from build123d import *

# Parameters (mm, degrees)
F0_R            = 50
F1_DEPTH        = 50
F2_R            = 25
F3_DEPTH        = 50
F5_DEPTH        = 50
F5_COPIES_COUNT = 12


# Not quite as in the source:
# - a pattern or mirror of a feature is missing from the dataset's text; its kind, count and spacing are read off the source's solid


with BuildPart() as f1:
    # F0 (on Top) → F1 (new body)
    with BuildSketch(Plane.XY):
        Circle(F0_R)
    extrude(amount=F1_DEPTH)

    # F2 (on Top) → F3 (cut)
    with BuildSketch(Plane.XY):
        Circle(F2_R)
    extrude(amount=F3_DEPTH, mode=Mode.SUBTRACT)

    # F4 (on Top) → F5 (join)
    with BuildSketch(Plane.XY):
        with BuildLine():
            Line((24.2363690546, 14.6788293603), (23.4842319041, 10.750179179))
            ThreePointArc((23.4842319041, 10.750179179), (35.7966783621, 13.5258846201), (42.1475842595, 24.4330782443))
            Line((42.1475842595, 24.4330782443), (38.1746449562, 24.8975734892))
            ThreePointArc((38.1746449562, 24.8975734892), (33.4316236094, 16.7517982205), (24.2363690546, 14.6788293603))
        make_face()
    f5 = extrude(amount=-F5_DEPTH)

    # F5_copies: F5 ×12 about axis
    f5_copies_axis = Axis((0, 0, 0), (0, 0, 1))
    for i in range(1, F5_COPIES_COUNT):
        add(f5.rotate(f5_copies_axis, i * 360 / F5_COPIES_COUNT))


solid = f1.part
Check sheet for the modelled part. Datum: model origin and axes. Units: mm. A direction names the side the tool comes from. Give positions to 0.01 mm unless a question says otherwise; leave off trailing zeros. Write each loop counter-clockwise with the first axis right and the second up, starting at its lowest first coordinate (ties: lowest second). Pieces come first, ordered by that corner, then holes. Notation, with made-up numbers: (3, 77) -> (9, 77) arc R19 ccw to (9, 112) -> close; hole circle Ø9 at (40.5, 50). An arc over 180 degrees is marked (long way). One line per item, written item: value. Start each with the question number.
Item 1: Section check C-C on z = -32. State how many separate pieces and enclosed holes the cut face has, then the cut area to 3 significant figures.
Item 2: Section check A-A on x = -16.5. Record the cut outline in (y, z), then the cut area to 3 significant figures.
Item 3: Draft check along X on faces 5 (the flat face through (-40.19, -24.66, -24.65)), 6 (the cylindrical face through (-20.63, -31.35, -24.65)), 7 (the flat face through (-33, -16, -50)), 8 (the cylindrical face through (-33.5, -16.8, -24.6)). Enter one of: +X half, -X half, draft (parallel to the pull), parting line (faces both ways), or undercut.
Item 4: Material ranges on probe 1 along Y at (x, z) = (0, 32); probe 2 along X at (y, z) = (-40, -3.5); probe 3 along Y at (x, z) = (-36, -37.5), recorded low to high. Write a range as from..to.
Item 5: Section check D-D on y = 30.5. Record the cut outline in (x, z), then the cut area to 3 significant figures.
Item 6: Tool access check on faces 1 (the flat face through (41.45, -22.47, -24.65)), 2 (the flat face through (-1.26, 47.14, -24.65)), 3 (the flat face through (47.14, 1.26, -24.65)), 4 (the cylindrical face through (29.446, -24.164, -24.65)). Record the directions out of +Z, -Z, +X, -X, +Y, -Y that give a thin tool (end or side, any length) a straight path to the whole face; none if there is none.
Item 7: Section check B-B on z = 32. Record the cut outline in (x, y), then the cut area to 3 significant figures.
Item 8: Gauge pin test, flat ends, axial feed: pin 1 (2 mm diameter, centred on x = -33, z = 11, fed in from +Y); pin 2 (5 mm diameter, centred on y = 11.5, z = -25.5, fed in from +X); pin 3 (5 mm diameter, centred on y = 27, z = -1, fed in from -X). Record the tip position at first contact, or that the pin passes through.
Results list:
1. separate pieces: 12
1. enclosed holes: 0
1. area: 1,090 mm²
2. outline: (-47.2, 0) -> (-26.28, 0) -> (-26.28, -50) -> (-21.68, -50) -> (-21.68, 0) -> (-18.78, 0) -> (-18.78, 50) -> (-47.2, 50) -> close; (18.78, 0) -> (33.07, 0) -> (33.07, -50) -> (38.87, -50) -> (38.87, 0) -> (47.2, 0) -> (47.2, 50) -> (18.78, 50) -> close
2. area: 3,360 mm²
3. face 5: -X half
3. face 6: undercut
3. face 7: draft
3. face 8: undercut
4. probe 1: -50..-25, 25..50
4. probe 2: -25.06..-20.87, -5.78..-1.6, 18.13..24.68
4. probe 3: -19.33..-13.68, 2.28..6.28, 21.58..25.58
5. outline: (-39.62, 0) -> (-15.18, 0) -> (-15.18, -50) -> (-10.99, -50) -> (-10.99, 0) -> (0.89, 0) -> (0.89, -50) -> (5.27, -50) -> (5.27, 0) -> (20.23, 0) -> (20.23, -50) -> (24.6, -50) -> (24.6, 0) -> (39.62, 0) -> (39.62, 50) -> (-39.62, 50) -> close
5. area: 4,610 mm²
6. face 1: -Z, +X
6. face 2: -Z, -X, +Y
6. face 3: -Z, +X, +Y
6. face 4: -Z
7. outline: circle Ø100 at (0, 0); hole circle Ø50 at (0, 0)
7. area: 5,890 mm²
8. pin 1: y = 38.42
8. pin 2: x = 36.41
8. pin 3: x = -43.47
